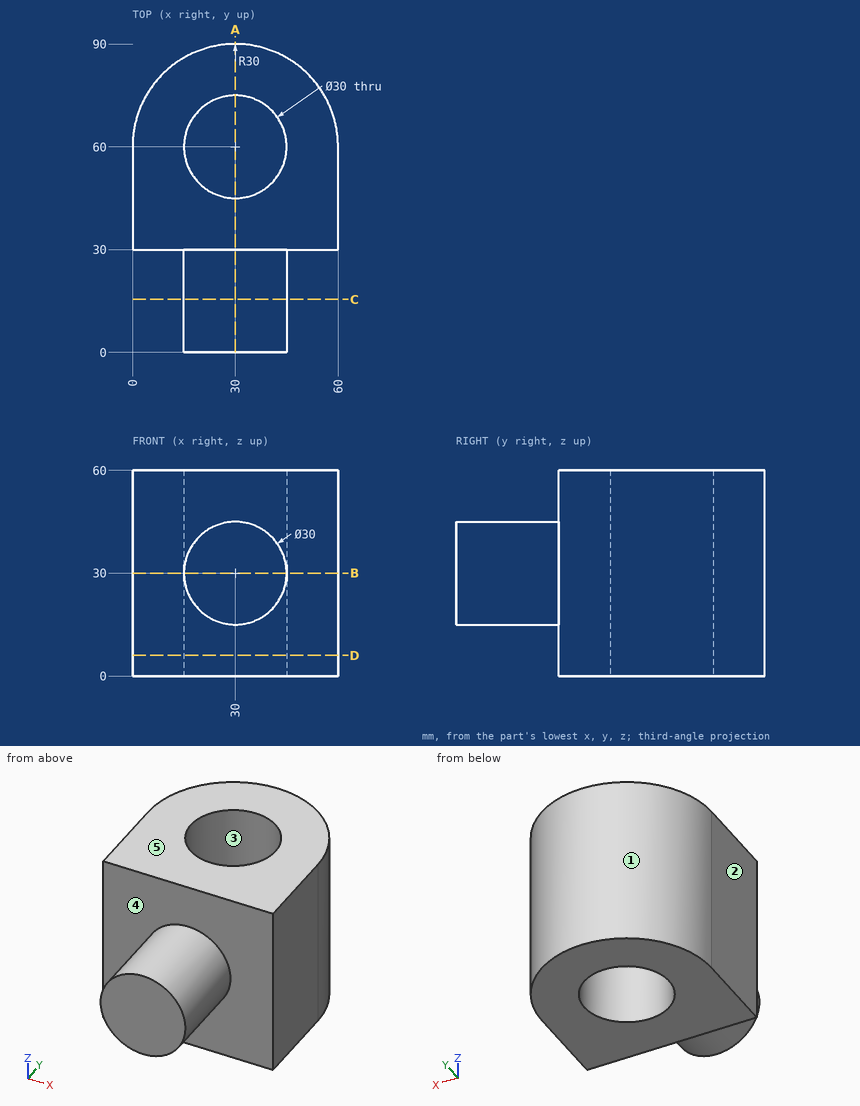
Geometry check sheet. Reference: drawing and pictorial views, mm from the part's lowest x, y, z. A direction names the side the tool comes from. Coordinates: 2 decimals unless noted, no trailing zeros. Write each loop counter-clockwise with the first axis right and the second up, starting at its lowest first coordinate (ties: lowest second). Pieces come first, ordered by that corner, then holes. Notation, with made-up numbers: M -15,-21 L 6,-21 A15 ccw 6,-6 Z; hole C 19.25,9.5 d4. An arc over 180 degrees is marked long. One line per question, with ' | ' between items.
1) Sectioned sample at A-A on x = 30. Record the cut outline in (y, z), then the cut area to 3 significant figures.
Solutions:
outline: M 0,15 L 30,15 L 30,0 L 45,0 L 45,60 L 30,60 L 30,45 L 0,45 Z; M 75,0 L 90,0 L 90,60 L 75,60 Z | area: 2,700 mm^2
2) Depth check by flat-ended pin: pin 1 Ø1.5 at (y, z) = (77, 10.5) entering from +X; pin 2 Ø12 at (y, z) = (78.5, 24) entering from -X; pin 3 Ø6 at (y, z) = (25.5, 40) entering from -X; pin 4 Ø5 at (x, z) = (38, 14.5) entering from -Y. Enter the tip coordinate at first touch or a pass-through.
Solutions:
pin 1: x = 55.22 | pin 2: x = 2.73 | pin 3: x = 16.73 | pin 4: y = 0
3) Sectioned sample at B-B on z = 30. Record the cut outline in (x, y), then the cut area to 3 significant figures.
Solutions:
outline: M 0,30 L 15,30 L 15,0 L 45,0 L 45,30 L 60,30 L 60,60 A30 ccw 0,60 Z; hole C 30,60 d30 | area: 3,410 mm^2
4) Release check for a two-part mould opening along X. For the marked faces 1, 2 and 3 record: +X half, -X half, draft (parallel to the pull), parting line (faces both ways), or undercut.
Solutions:
face 1: parting line | face 2: -X half | face 3: undercut
5) Material ranges on L1, parallel to Y at x = 30, z = 20; L2, parallel to Y at x = 41, z = 57.5; L3, parallel to Y at x = 2.5, z = 20.5, recorded low to high.
Solutions:
L1: 0 to 45, 75 to 90 | L2: 30 to 49.8, 70.2 to 87.91 | L3: 30 to 71.99
6) Access from +Z, -Z, +X, -X, +Y, -Y to the whole of each face (thin tool, end or side, straight path). Record for the marked faces 4 and 5.
Solutions:
face 4: -Y | face 5: +Z, +X, -X, +Y, -Y
7) Sectioned sample at C-C on y = 15.5. Record the cut outline in (x, z), then the cut area to 3 significant figures.
Solutions:
outline: C 30,30 d30 | area: 707 mm^2
8) Sectioned sample at D-D on z = 6. Record the cut outline in (x, y), then the cut area to 3 significant figures.
Solutions:
outline: M 0,30 L 60,30 L 60,60 A30 ccw 0,60 Z; hole C 30,60 d30 | area: 2,510 mm^2
